Input: part model. Units: mm. Frame: model coordinates. Give positions to 0.01 mm unless a question says otherwise; leave off trailing zeros. Loops run counter-clockwise (first coordinate to the right, second up) from the corner with the lowest first, then second, coordinate; pieces in that order, holes last. Notation, with made-up numbers: (18.25, 29) -> (36.25, 29) arc R17 cw to (36.25, 37) -> close; hole circle Ø5 at (86.5, -33). An arc over 180 degrees is marked (long way). Use CSV: the item, a comma, the result in double quotes.
```python
from build123d import *

# Parameters (mm, degrees)
SKETCH1_W           = 152.4
SKETCH1_H           = 19.05
BOSS_EXTRUDE1_DEPTH = 3.175
FILLET1_R           = 6.35
SKETCH2_R           = 3.175
SKETCH2_R_2         = 3.81
CUT_EXTRUDE1_DEPTH  = 100.507657605


with BuildPart() as part:
    # Sketch1 → Boss-Extrude1 (new body)
    with BuildSketch(Plane(origin=(0, 0, 0), x_dir=(1, 0, 0), z_dir=(0, 1, 0))):
        with Locations((21.802018925, 7.424854969)):
            Rectangle(SKETCH1_W, SKETCH1_H)
    extrude(amount=BOSS_EXTRUDE1_DEPTH)

    # Fillet1
    fillet1_edges = [part.edges().sort_by_distance(p)[0] for p in [
        (-54.397981075, 1.5875, -16.949854969),
        (98.002018925, 1.5875, -16.949854969),
        (98.002018925, 1.5875, 2.100145031),
        (-54.397981075, 1.5875, 2.100145031),
    ]]
    fillet(fillet1_edges, radius=FILLET1_R)

    # Sketch2 → Cut-Extrude1 (cut, through all)
    with BuildSketch(Plane(origin=(0, 3.175, 0), x_dir=(1, 0, 0), z_dir=(0, 1, 0))):
        with Locations(Location((-48.047981075, 7.424854969, 0), (0, 0, 270))):
            Circle(SKETCH2_R)
        with Locations(Location((-35.347981075, 7.424854969, 0), (0, 0, 270))):
            Circle(SKETCH2_R)
        with Locations(Location((80.222018925, 7.424854969, 0), (0, 0, 270))):
            Circle(SKETCH2_R_2)
        with BuildLine():
            Line((87.842018925, 8.377354969), (92.922018925, 8.377354969))
            ThreePointArc((92.922018925, 8.377354969), (93.874518925, 7.424854969), (92.922018925, 6.472354969))
            Line((92.922018925, 6.472354969), (87.842018925, 6.472354969))
            ThreePointArc((87.842018925, 6.472354969), (86.889518925, 7.424854969), (87.842018925, 8.377354969))
        make_face()
        with BuildLine():
            Line((72.602018925, 6.408854969), (67.522018925, 6.408854969))
            ThreePointArc((67.522018925, 6.408854969), (66.506018925, 7.424854969), (67.522018925, 8.440854969))
            Line((67.522018925, 8.440854969), (72.602018925, 8.440854969))
            ThreePointArc((72.602018925, 8.440854969), (73.618018925, 7.424854969), (72.602018925, 6.408854969))
        make_face()
    extrude(amount=-CUT_EXTRUDE1_DEPTH, mode=Mode.SUBTRACT)


solid = part.part
```
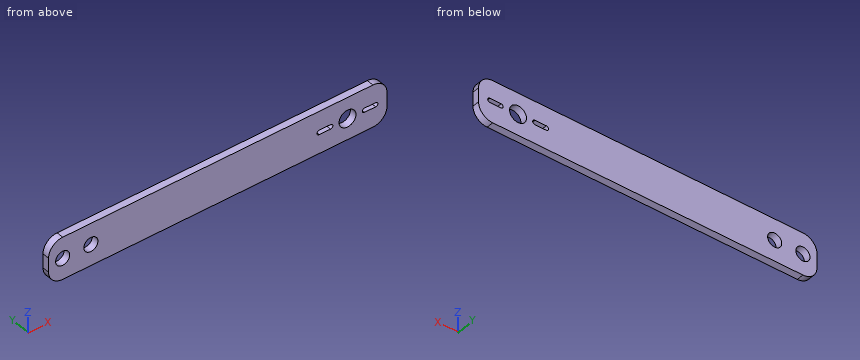
1) Ray query, line 1 (X direction, y = 2.2, z = -5.75); line 2 (X direction, y = 1.1, z = -10); line 3 (X direction, y = 2.8, z = -7). Return the intervals inside material, ascending.
From the geometry:
line 1,"x = -54.4 to -50.75, -45.35 to -38.05, -32.65 to 76.8, 83.64 to 98"
line 2,"x = -54.4 to -49.91, -46.19 to -37.21, -33.49 to 77.41, 83.03 to 98"
line 3,"x = -54.4 to -51.19, -44.9 to -38.49, -32.2 to 66.6, 73.52 to 76.44, 84.01 to 86.99, 93.77 to 98"
2) Contact query for a flat-ended pin moving along its axis: pin 1 (5.5 mm diameter, centred on x = -48.05, z = -7.42, fed in from -Y). Output: stop coordinate, or through.
From the geometry:
pin 1,"passes through"
3) Section query A-A (x = 70). Return loops of the section in (y, z) (3 decimals), then the cut area to 3 significant figures.
From the geometry:
outline,"(0, -16.95) -> (3.175, -16.95) -> (3.175, -8.441) -> (0, -8.441) -> close; (0, -6.409) -> (3.175, -6.409) -> (3.175, 2.1) -> (0, 2.1) -> close"
area,"54.0 mm^2"
4) Section query B-B (y = 1.05). Give the number of separate pieces and of enclosed holes in the cut face, then the cut area to 3 significant figures.
From the geometry:
separate pieces,"1"
enclosed holes,"5"
area,"2,730 mm^2"
5) Section query D-D (z = -15). Return loops of the section in (x, y) (3 decimals), then the cut area to 3 significant figures.
From the geometry:
outline,"(-52.626, 0) -> (96.23, 0) -> (96.23, 3.175) -> (-52.626, 3.175) -> close"
area,"473 mm^2"
6) Section query C-C (z = 0.75). Return loops of the section in (x, y) (3 decimals), then the cut area to 3 significant figures.
From the geometry:
outline,"(-51.963, 0) -> (95.567, 0) -> (95.567, 3.175) -> (-51.963, 3.175) -> close"
area,"468 mm^2"
